Read the model definition and answer for the solid it produces. Units are mm, in the model's axes. Coordinates: 2 decimals unless noted, no trailing zeros. Order: outer loops, then holes, each group sorted by start corner. A loop starts at its lowest first (then second) coordinate and runs counter-clockwise, first axis right, second up. Notation, with made-up numbers: (3, 33.25) -> (25, 33.25) arc R18 cw to (25, 57.25) -> close; hole circle Ø2 at (46.25, 58.5). An arc over 180 degrees is marked (long way). Answer as a JSON object with one key per item and string values. Group by question number.
1) Section A-A on x = 5.5 is taken. Determine the outline of the cut face in (y, z).
2) Section C-C on z = 3.05 is taken. Count the separate pieces of the cut face and the enclosed holes in it, and give its area (3 significant figures).
3) Consider L1, parallel to X at y = 53, z = 0.35; L2, parallel to Y at x = 106, z = 4.3. Determine where each line is inside the solid, lowest interval first.
4) Given pin 1 (6 mm diameter, centred on x = 110, y = 45, fed in from -Z), flat-ended and moving along its own axis, determine where the tip first touches the part or whether it passes through.
from build123d import *

# Parameters (mm, degrees)
SKETCH1_W           = 190
SKETCH1_H           = 190
BOSS_EXTRUDE1_DEPTH = 5
SKETCH2_R           = 2.5
CUT_EXTRUDE1_DEPTH  = 177.847391838
LPATTERN1_COUNT     = 6
LPATTERN1_PITCH     = 30


with BuildPart() as part:
    # Sketch1 → Boss-Extrude1 (new body)
    with BuildSketch(Plane.XY):
        with BuildLine():
            Line((-105, 125), (105, 125))
            ThreePointArc((105, 125), (119.142135624, 119.142135624), (125, 105))
            Line((125, 105), (125, -105))
            ThreePointArc((125, -105), (119.142135624, -119.142135624), (105, -125))
            Line((105, -125), (-105, -125))
            ThreePointArc((-105, -125), (-119.142135624, -119.142135624), (-125, -105))
            Line((-125, -105), (-125, 105))
            ThreePointArc((-125, 105), (-119.142135624, 119.142135624), (-105, 125))
        make_face()
        Rectangle(SKETCH1_W, SKETCH1_H, mode=Mode.SUBTRACT)
    extrude(amount=BOSS_EXTRUDE1_DEPTH)

    # Sketch2 → Cut-Extrude1 (cut, through all)
    with BuildSketch(Plane.XY.offset(5)):
        with Locations((-110, 75)):
            Circle(SKETCH2_R)
        with Locations((110, 75)):
            Circle(SKETCH2_R)
    cut_extrude1 = extrude(amount=-CUT_EXTRUDE1_DEPTH, mode=Mode.SUBTRACT)

    # LPattern1: Cut-Extrude1 ×6
    with Locations(*[(0, -i * LPATTERN1_PITCH, 0) for i in range(1, LPATTERN1_COUNT)]):
        add(cut_extrude1, mode=Mode.SUBTRACT)


solid = part.part
Worked answers:
{
 "1": {"outline": "(-125, 0) -> (-95, 0) -> (-95, 5) -> (-125, 5) -> close; (95, 0) -> (125, 0) -> (125, 5) -> (95, 5) -> close"},
 "2": {"separate pieces": "1", "enclosed holes": "13", "area": "25,800 mm²"},
 "3": {"L1": "x = -125 to -95, 95 to 125", "L2": "y = -124.97 to 124.97"},
 "4": {"pin 1": "stops at z = 0"}
}
